The listing builds one solid part. Answer for the finished solid, in the listing's coordinates (mm). Face numbers are marked on the shaded views. A direction names the side the tool comes from. Round coordinates to 2 decimals unless told otherwise and drop trailing zeros. Write each loop counter-clockwise with the first axis right and the second up, starting at its lowest first coordinate (ties: lowest second). Pieces come first, ordered by that corner, then holes. Notation, with made-up numbers: (50.5, 31.5) - (70.5, 31.5) arc R10 cw to (70.5, 45.5) - close; hole circle Ø5 at (75.25, 17). An arc over 180 degrees is marked (long way). Return JSON: item names as keys, results as strings. Group by question number.
(1) Section B-B, the plane z = 46.5 is taken. Write down the section's boundary in (x, y).
(2) Section A-A, the plane z = 10 is taken. Write down the section's boundary in (x, y), then the cut area to 3 significant figures.
(3) Which of the six approach directions +Z, -Z, +X, -X, +Y, -Y give full straight-line access (tool end or side, diameter ignored) to the marked faces 1 and 2?
(4) Find the intervals of material crossed by line 1 along X through (y, z) = (0, 3.5); line 2 along Y through (x, z) = (0, 4.75); line 3 along Z through (x, y) = (-3.5, -1.25), in increasing order. Write a range as [from, to].
(5) Each of these flat-tipped pins is pushed along its axis until it touches: pin 1 (3.5 mm diameter, centred on x = -0.5, z = 7.5, fed in from +Y); pin 2 (6.5 mm diameter, centred on x = 0, y = 0, fed in from -Z); pin 3 (1 mm diameter, centred on x = -1, z = 58, fed in from +Y); pin 4 (2 mm diameter, centred on x = -0.5, y = 3.5, fed in from +Z). Where does it stop, or does it pass through?
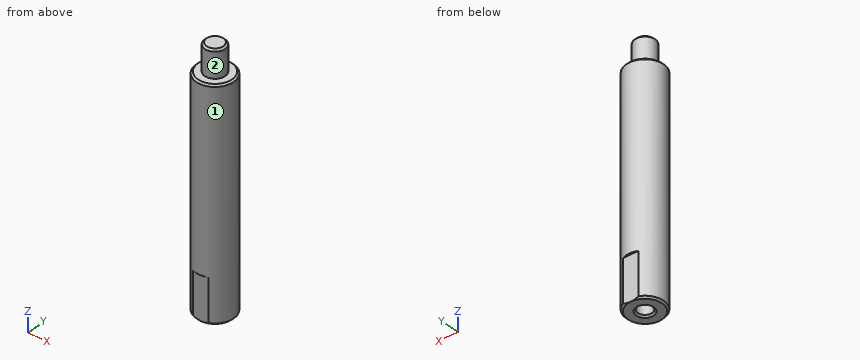
```python
from build123d import *

# Parameters (mm, degrees)
SKETCH_1_R             = 5.5
EXTRUDE_1_DEPTH        = 66
CHAMFER_1_SIZE         = 0.5
SKETCH_2_R             = 3.3
EXTRUDE_2_DEPTH        = 8
HOLE_WIZARD_M5_1_D     = 4.2
HOLE_WIZARD_M5_1_DEPTH = 12.4
HOLE_WIZARD_M5_1_TIP   = 1.2618073
CHAMFER_3_SIZE         = 0.5
SKETCH_6_W             = 10
SKETCH_6_H             = 3
CUT_EXTRUDE_1_DEPTH    = 13


# Read off the part's stored shape, not the designer's step: M6 机械螺纹 螺柱1
with BuildPart() as part:
    # 草图1 → 拉伸1 (new body)
    with BuildSketch(Plane.XY):
        Circle(SKETCH_1_R)
    extrude(amount=EXTRUDE_1_DEPTH)

    # 倒角1
    chamfer_1_edges = [part.edges().sort_by_distance(p)[0] for p in [
        (-5.5, 0, 0),
        (-5.5, 0, 66),
    ]]
    chamfer(chamfer_1_edges, length=CHAMFER_1_SIZE)

    # 草图2 → 拉伸2 (add)
    with BuildSketch(Plane.XY.offset(66)):
        Circle(SKETCH_2_R)
    extrude(amount=EXTRUDE_2_DEPTH)

    # M5 螺纹孔1
    with Locations(Plane(origin=(0, 0, 0), x_dir=(-1, 0, 0), z_dir=(0, 0, -1))):
        with Locations((0, 0)):
            Hole(HOLE_WIZARD_M5_1_D / 2, depth=HOLE_WIZARD_M5_1_DEPTH)
            with Locations((0, 0, -(HOLE_WIZARD_M5_1_DEPTH + HOLE_WIZARD_M5_1_TIP / 2))):  # 118° drill point
                Cone(0, HOLE_WIZARD_M5_1_D / 2, HOLE_WIZARD_M5_1_TIP, mode=Mode.SUBTRACT)

    # 倒角3
    chamfer_3_edges = [part.edges().sort_by_distance(p)[0] for p in [
        (-2.1, 0, 0),
    ]]
    chamfer(chamfer_3_edges, length=CHAMFER_3_SIZE)

    # 草图6 → 切除-拉伸1 (cut)
    with BuildSketch(Plane(origin=(0, 0, 0), x_dir=(-1, 0, 0), z_dir=(0, 0, -1))):
        with Locations((0, 6.5)):
            Rectangle(SKETCH_6_W, SKETCH_6_H)
        with Locations((0, -6.5)):
            Rectangle(SKETCH_6_W, SKETCH_6_H)
    extrude(amount=-CUT_EXTRUDE_1_DEPTH, mode=Mode.SUBTRACT)

    # M6 机械螺纹 螺柱1 outline → M6 机械螺纹 螺柱1 (revolve, cut)
    with BuildSketch(Plane.XZ):
        Polygon((3.3, 74), (2.4585, 74), (3, 73.4585), (3, 66), (3.3, 66), align=None)
    revolve(axis=Axis((0, 0, 0), (0, 0, 1)), mode=Mode.SUBTRACT)


solid = part.part
```
Working result:
{
 "1": {"outline": "circle Ø11 at (0, 0)"},
 "2": {"outline": "(-2.29, -5) - (2.29, -5) arc R5.5 ccw to (2.29, 5) - (-2.29, 5) arc R5.5 ccw to start; hole circle Ø4.2 at (0, 0)", "area": "78.1 mm^2"},
 "3": {"face 1": "+Z, -Z", "face 2": "+Z"},
 "4": {"line 1": "x = [-5.5, -2.1], [2.1, 5.5]", "line 2": "y = [-5, -2.1], [2.1, 5]", "line 3": "z = [0, 66]"},
 "5": {"pin 1": "stops at y = 5", "pin 2": "stops at z = 0", "pin 3": "stops at y = 5.48", "pin 4": "stops at z = 73.92"}
}
